from build123d import *

# Parameters (mm, degrees)
BOSS_EXTRU_1_DEPTH            = 50
CONG_4_R                      = 35
CONG_5_R                      = 35
CONG_6_R                      = 30
CONG_12_R                     = 10
ESQUISSE3_R                   = 11
ENL_V_MAT_EXTRU_4_DEPTH       = 50
ENL_V_MAT_EXTRU_8_DEPTH       = 251
ESQUISSE6_R                   = 2
ENL_V_MAT_EXTRU_9_DEPTH       = 58
ENL_V_MAT_EXTRU_12_DEPTH      = 251.898527225
ENL_V_MAT_EXTRU_12_DEPTH_BACK = 179
ESQUISSE11_R                  = 3
ENL_V_MAT_EXTRU_14_DEPTH      = 20
BOSS_EXTRU_2_DEPTH            = 5


with BuildPart() as part:
    # Esquisse1 → Boss.-Extru.1 (new body)
    with BuildSketch(Plane.XY):
        Polygon((-129.391143911, 131.10701107), (-129.391143911, -98.89298893), (-124.391143911, -98.89298893), (-124.391143911, -33.89298893), (-64.391143911, -33.89298893), (-64.391143911, -98.89298893), (-49.391143911, -98.89298893), (-49.391143911, 131.10701107), align=None)
    extrude(amount=BOSS_EXTRU_1_DEPTH)

    # Congé4
    cong_4_edges = [part.edges().sort_by_distance(p)[0] for p in [
        (-129.391143911, 16.10701107, 50),
    ]]
    fillet(cong_4_edges, radius=CONG_4_R)

    # Congé5
    # the kernel refuses this fillet: 35 mm, written as the material it takes off along each edge
    with BuildSketch(Plane(origin=(-129.391143911, 202.914044152, 0), x_dir=(0, 0, 1), z_dir=(0, -1, 0))) as cong_5_piece_1:
        with BuildLine():
            CenterArc((35, -28.722813233), CONG_5_R, 124.849904579, 55.150095421)
            Line((0, -28.722813233), (-0.7, -28.722813233))
            Line((-0.7, -28.722813233), (-0.7, 0))
            Line((-0.7, 0), (0, 0.7))
            ThreePointArc((0, 0.7), (7.5, 0.7), (14.6, 0.574456265))
            Line((14.6, 0.574456265), (15, 0))
        make_face()
    extrude(amount=373.614066163, mode=Mode.SUBTRACT)

    # Congé6
    # the kernel refuses this fillet: 30 mm, written as the material it takes off along each edge
    with BuildSketch(Plane(origin=(-49.391143911, -173.89298893, 0), x_dir=(-1, 0, 0), z_dir=(0, 1, 0))) as cong_6_piece_1:
        with BuildLine():
            CenterArc((CONG_6_R, CONG_6_R), CONG_6_R, 180, 90)
            Line((0, CONG_6_R), (0, 0))
            Line((0, 0), (CONG_6_R, 0))
        make_face()
    extrude(amount=380, mode=Mode.SUBTRACT)
    with BuildSketch(Plane(origin=(-49.391143911, -173.89298893, 50), x_dir=(-1, 0, 0), z_dir=(0, 1, 0))) as cong_6_piece_2:
        with BuildLine():
            CenterArc((CONG_6_R, -CONG_6_R), CONG_6_R, 90, 90)
            Line((0, -CONG_6_R), (0, 0))
            Line((0, 0), (CONG_6_R, 0))
        make_face()
    extrude(amount=380, mode=Mode.SUBTRACT)

    # Congé12
    cong_12_edges = [part.edges().sort_by_distance(p)[0] for p in [
        (-124.391143911, -33.89298893, 21.146981396),
        (-64.391143911, -33.89298893, 25),
    ]]
    fillet(cong_12_edges, radius=CONG_12_R)

    # Esquisse3 → Enlèv. mat.-Extru.4 (cut)
    with BuildSketch(Plane.ZY.offset(64.391143911)):
        with Locations(Location((25, -81.917553746, 0), (0, 0, 270))):
            Circle(ESQUISSE3_R)
    extrude(amount=-ENL_V_MAT_EXTRU_4_DEPTH, mode=Mode.SUBTRACT)

    # Esquisse5 → Enlèv. mat.-Extru.8 (cut)
    with BuildSketch(Plane(origin=(0, 131.10701107, 0), x_dir=(1, 0, 0), z_dir=(0, 1, 0))):
        with BuildLine():
            Line((-86.891143911, -50), (-86.891143911, 0))
            ThreePointArc((-86.891143911, 0), (-162.141280076, -25), (-86.891143911, -50))
        make_face()
    extrude(amount=-ENL_V_MAT_EXTRU_8_DEPTH, mode=Mode.SUBTRACT)

    # Esquisse6 → Enlèv. mat.-Extru.9 (cut)
    with BuildSketch(Plane.ZY.offset(86.891143911)):
        with Locations((7.5, 98.60701107)):
            Circle(ESQUISSE6_R)
        with Locations((42.5, 98.60701107)):
            Circle(ESQUISSE6_R)
        with Locations((42.5, -1.39298893)):
            Circle(ESQUISSE6_R)
        with Locations((7.5, -1.39298893)):
            Circle(ESQUISSE6_R)
    extrude(amount=-ENL_V_MAT_EXTRU_9_DEPTH, mode=Mode.SUBTRACT)

    # Esquisse9 → Enlèv. mat.-Extru.12 (cut, two sides: drawn at the far end of the back side and taken through both)
    with BuildSketch(Plane(origin=(0, 131.10701107, 0), x_dir=(1, 0, 0), z_dir=(0, 1, 0)).offset(-ENL_V_MAT_EXTRU_12_DEPTH_BACK)):
        with BuildLine():
            Line((-195.505666121, -17.5), (-86.891143911, -17.5))
            ThreePointArc((-86.891143911, -17.5), (-79.391143911, -25), (-86.891143911, -32.5))
            Line((-86.891143911, -32.5), (-195.505666121, -32.5))
            Line((-195.505666121, -32.5), (-412.73471054, -32.5))
            Line((-412.73471054, -32.5), (-412.73471054, -17.5))
            Line((-412.73471054, -17.5), (-195.505666121, -17.5))
        make_face()
    extrude(amount=ENL_V_MAT_EXTRU_12_DEPTH + ENL_V_MAT_EXTRU_12_DEPTH_BACK, mode=Mode.SUBTRACT)

    # Esquisse11 → Enlèv. mat.-Extru.14 (cut)
    with BuildSketch(Plane.ZY.offset(49.810744996)):
        with Locations(Location((42.5, 98.60701107, 0), (0, 0, 180))):
            Circle(ESQUISSE11_R)
        with Locations(Location((7.5, 98.60701107, 0), (0, 0, 180))):
            Circle(ESQUISSE11_R)
        with Locations(Location((42.5, -1.39298893, 0), (0, 0, 180))):
            Circle(ESQUISSE11_R)
        with Locations(Location((7.5, -1.39298893, 0), (0, 0, 180))):
            Circle(ESQUISSE11_R)
    extrude(amount=ENL_V_MAT_EXTRU_14_DEPTH, mode=Mode.SUBTRACT)

    # Esquisse12 → Boss.-Extru.2 (add)
    with BuildSketch(Plane(origin=(0, 131.10701107, 0), x_dir=(1, 0, 0), z_dir=(0, 1, 0))):
        with BuildLine():
            Line((-79.391143911, 0), (-86.891143911, 0))
            Line((-86.891143911, 0), (-86.891143911, -17.5))
            ThreePointArc((-86.891143911, -17.5), (-79.391143911, -25), (-86.891143911, -32.5))
            Line((-86.891143911, -32.5), (-86.891143911, -50))
            Line((-86.891143911, -50), (-79.391143911, -50))
            ThreePointArc((-79.391143911, -50), (-60.02622718, -42.912878475), (-49.810744996, -25))
            ThreePointArc((-49.810744996, -25), (-60.02622718, -7.087121525), (-79.391143911, 0))
        make_face()
    extrude(amount=BOSS_EXTRU_2_DEPTH)


solid = part.part
For this review, take the finished solid that the model builds, in its own axes (mm). A direction names the side the tool comes from. Round coordinates to 2 decimals unless told otherwise and drop trailing zeros. Loops run counter-clockwise (first coordinate to the right, second up) from the corner with the lowest first, then second, coordinate; pieces in that order, holes last. Notation, with made-up numbers: (-8, 58) - (49, 58) arc R14 ccw to (49, 77) - close; hole circle Ø1 at (-12, 21.25). An arc over 180 degrees is marked (long way). Put each result on its own line as item: value. Start each with the question number.
1. Insertion check: P1, Ø1.5, axis at x = -54.5, y = -41, coming from the +Z side; P2, Ø5, axis at y = -3, z = 43, coming from the +X side; P3, Ø21, axis at y = -76.5, z = 24, coming from the -X side; P4, Ø2.5, axis at y = 98.61, z = 7.5, coming from the -X side. Each pin has a flat end and moves straight along its axis. Give the tip position at first contact, or say it passes through.
2. For faces 4 (the flat face through (-64.391, -65, 25)), 5 (the flat face through (-69, 136.107, 25)), 6 (the flat face through (-69.811, 101, 7)), list the 3-axis set-ups (+Z, -Z, +X, -X, +Y, -Y) from which the entire face can be reached by the end or side of a thin tool; tool diameter is ignored.
3. Consider section B-B on z = 29. State the section outline as (x, y) points.
4. Consider section A-A on z = 7.5. State the section outline as (x, y) points, plus the area to 3 significant figures.
5. Consider section C-C on x = -54.5. State the section outline as (y, z) points, plus the area to 3 significant figures.
6. Mouldability with a two-part tool opening along Y and no side actions: class faces 1 (the cylindrical face through (-67.398, -36.745, 25.344)), 2 (the flat face through (-83, 50, 50)), 3 (the flat face through (-69.811, 1, 42)) as +Y half, -Y half, draft (parallel to the pull), parting line (faces both ways), or undercut.
7. For probe 1 along Y at (x, z) = (-64, 26); probe 2 along Y at (x, z) = (-73, 42); probe 3 along Y at (x, z) = (-61.5, 23.5), list the stretches that pass through material, from the lowest coordinate up. Write a range as [from, to].
Result sheet:
1. P1: z = 37.81
1. P2: x = -57.59
1. P3: x = -64.39
1. P4: through
2. face 4: +Z, -Z, -X, -Y
2. face 5: +Z, -Z, +X, -X, +Y
2. face 6: +X
3. outline: (-80.55, -33.89) - (-74.39, -33.89) arc R10 cw to (-64.39, -43.89) - (-64.39, -71.67) - (-50.77, -71.67) - (-50.77, 136.11) - (-80.55, 136.11) - close; (-64.39, -98.89) - (-50.77, -98.89) - (-50.77, -92.16) - (-64.39, -92.16) - close
4. outline: (-86.89, -33.89) - (-74.39, -33.89) arc R10 cw to (-64.39, -43.89) - (-64.39, -98.89) - (-59.55, -98.89) - (-59.55, -4.39) - (-69.81, -4.39) - (-69.81, -3.39) - (-86.89, -3.39) - close; (-86.89, 0.61) - (-69.81, 0.61) - (-69.81, 1.61) - (-59.55, 1.61) - (-59.55, 95.61) - (-69.81, 95.61) - (-69.81, 96.61) - (-86.89, 96.61) - close; (-86.89, 100.61) - (-69.81, 100.61) - (-69.81, 101.61) - (-59.55, 101.61) - (-59.55, 136.11) - (-86.89, 136.11) - close
4. area: 4,720 mm^2
5. outline: (-98.89, 13.25) - (136.11, 13.25) - (136.11, 36.75) - (-98.89, 36.75) - close; hole circle Ø22 at (-81.92, 25)
5. area: 5,140 mm^2
6. face 1: -Y half
6. face 2: draft
6. face 3: undercut
7. probe 1: [-98.89, -92.87], [-70.96, 136.11]
7. probe 2: [-33.99, -3.33], [0.54, 96.67], [100.54, 136.11]
7. probe 3: [-98.89, -92.81], [-71.02, 136.11]
